```python
from build123d import *

# Parameters (mm, degrees)
MODEL_R             = 0.5842
MODEL_R_2           = 1.5748
BOSS_EXTRUDE1_DEPTH = 1.5748


with BuildPart() as part:
    # Model → Boss-Extrude1 (new body)
    with BuildSketch(Plane.XY):
        Polygon((0, 11.43), (1.27, 12.7), (26.67, 12.7), (27.94, 11.43), (27.94, 1.27), (26.67, 0), (1.27, 0), (0, 1.27), align=None)
        with Locations((10.795, 6.35)):
            Circle(MODEL_R, mode=Mode.SUBTRACT)
        with Locations((17.145, 6.35)):
            Circle(MODEL_R, mode=Mode.SUBTRACT)
        with Locations((3.81, 6.35)):
            Circle(MODEL_R_2, mode=Mode.SUBTRACT)
        with Locations((24.13, 6.35)):
            Circle(MODEL_R_2, mode=Mode.SUBTRACT)
        with Locations((13.335, 3.175)):
            Circle(MODEL_R, mode=Mode.SUBTRACT)
        with Locations((14.605, 9.525)):
            Circle(MODEL_R, mode=Mode.SUBTRACT)
    extrude(amount=BOSS_EXTRUDE1_DEPTH)


solid = part.part
```
Could you check a few things on this model? Use its own coordinates, in mm. Round coordinates to 2 decimals unless told otherwise and drop trailing zeros. Loops run counter-clockwise (first coordinate to the right, second up) from the corner with the lowest first, then second, coordinate; pieces in that order, holes last. Notation, with made-up numbers: M -23,70.5 L 27,70.5 A17 cw 27,77.5 Z; hole C 83,86 d8. An arc over 180 degrees is marked long. Put each result on its own line as item: value.
Q1. For pin 1 (0.9 mm diameter, centred on x = 17.145, y = 6.35, fed in from +Z), with a flat end and sliding along its axis, tell me the tip position at first contact or that it passes through.
Check result:
pin 1: through
Q2. Thinking about a two-plate mould opening in X: for faces 1 (the face through (14, 12.7, 1)), 2 (the face through (27.3, 12.07, 0.78)), 3 (the face through (16.681, 5.995, 0.776)), which applies, released by +X, released by -X, zero draft, split by the parting line, or undercut?
Check result:
face 1: zero draft
face 2: released by +X
face 3: undercut
Q3. Imagine slicing it at B-B (y = 6.35). Write out the boundary of the cut face in (x, z), then the cut area to 3 significant figures.
Check result:
outline: M 0,0 L 2.24,0 L 2.24,1.57 L 0,1.57 Z; M 5.38,0 L 10.21,0 L 10.21,1.57 L 5.38,1.57 Z; M 11.38,0 L 16.56,0 L 16.56,1.57 L 11.38,1.57 Z; M 17.73,0 L 22.56,0 L 22.56,1.57 L 17.73,1.57 Z; M 25.7,0 L 27.94,0 L 27.94,1.57 L 25.7,1.57 Z
area: 30.4 mm2
Q4. Imagine slicing it at C-C (y = 9.25). Write out the boundary of the cut face in (x, z), then the cut area to 3 significant figures.
Check result:
outline: M 0,0 L 14.09,0 L 14.09,1.57 L 0,1.57 Z; M 15.12,0 L 27.94,0 L 27.94,1.57 L 15.12,1.57 Z
area: 42.4 mm2
Q5. I need wall thicknesses on probe 1 along Y at (x, z) = (24.13, 1.05); probe 2 along X at (y, z) = (6.5, 0.25); probe 3 along X at (y, z) = (6, 1.05). Which ranges of each line are inside material? Lowest first, please.
Check result:
probe 1: 0 to 4.78, 7.92 to 12.7
probe 2: 0 to 2.24, 5.38 to 10.23, 11.36 to 16.58, 17.71 to 22.56, 25.7 to 27.94
probe 3: 0 to 2.27, 5.35 to 10.33, 11.26 to 16.68, 17.61 to 22.59, 25.67 to 27.94
Q6. Imagine slicing it at A-A (x = 3.81). Write out the boundary of the cut face in (y, z).
Check result:
outline: M 0,0 L 4.78,0 L 4.78,1.57 L 0,1.57 Z; M 7.92,0 L 12.7,0 L 12.7,1.57 L 7.92,1.57 Z
Q7. Imagine slicing it at D-D (z = 0.3). Write out the boundary of the cut face in (x, y) (3 decimals), then the cut area to 3 significant figures.
Check result:
outline: M 0,1.27 L 1.27,0 L 26.67,0 L 27.94,1.27 L 27.94,11.43 L 26.67,12.7 L 1.27,12.7 L 0,11.43 Z; hole C 3.81,6.35 d3.15; hole C 10.795,6.35 d1.168; hole C 13.335,3.175 d1.168; hole C 14.605,9.525 d1.168; hole C 17.145,6.35 d1.168; hole C 24.13,6.35 d3.15
area: 332 mm2
